Read the model definition and answer for the solid it produces. Units are mm, in the model's axes. A direction names the side the tool comes from. Coordinates: 2 decimals unless noted, no trailing zeros. Write each loop counter-clockwise with the first axis right and the second up, starting at its lowest first coordinate (ties: lowest second). Pieces come first, ordered by that corner, then holes. Notation, with made-up numbers: M 34.25,9 L 39.25,9 A16 cw 39.25,28 Z; hole C 41.25,-32.5 d4. An arc over 180 degrees is marked long. Use a Markdown table: item, result. Add a question column.
from build123d import *

# Parameters (mm, degrees)
SKETCH_1_W                  = 80
SKETCH_1_H                  = 83
EXTRUDE_1_DEPTH             = 12
HOLE_WIZARD_1_D             = 9
HOLE_WIZARD_1_CBORE_D       = 15
HOLE_WIZARD_1_CBORE_DEPTH   = 8
HOLE_WIZARD_1_2_D           = 46
HOLE_WIZARD_M6_2_D          = 5
HOLE_WIZARD_M6_1_AT_2_COUNT = 2
HOLE_WIZARD_M6_1_AT_2_PITCH = 15
CHAMFER_1_SIZE              = 1


with BuildPart() as part:
    # 草图1 → 凸台-拉伸1 (new body)
    with BuildSketch(Plane(origin=(0, 0, 0), x_dir=(0, 0, -1), z_dir=(1, 0, 0))):
        Rectangle(SKETCH_1_W, SKETCH_1_H)
    extrude(amount=EXTRUDE_1_DEPTH)

    # Hole Wizard 1 (through all)
    with Locations(Plane.ZY):
        with Locations((-25, 33.5), (25, 33.5)):
            CounterBoreHole(HOLE_WIZARD_1_D / 2, HOLE_WIZARD_1_CBORE_D / 2, HOLE_WIZARD_1_CBORE_DEPTH)

    # Hole Wizard 1 2 (through all)
    with Locations(Plane(origin=(12, 0, 0), x_dir=(0, 0, -1), z_dir=(1, 0, 0))):
        with Locations((0, -16.5)):
            Hole(HOLE_WIZARD_1_2_D / 2)

    # M6 螺纹孔2 (through all)
    with Locations(Plane.ZY):
        with Locations((-30, -16.5), (30, -16.5)):
            Hole(HOLE_WIZARD_M6_2_D / 2)

    # 草图8 → M6 螺纹孔1 (revolve, cut)
    with BuildSketch(Plane(origin=(6, -9, -40), x_dir=(0, 1, 0), z_dir=(1, 0, 0))):
        Polygon((0, 0), (0, 16.502151548), (2.5, 15), (2.5, 0), align=None)
    hole_wizard_m6_1 = revolve(axis=Axis((6, -9, -46.35), (0, 0, 1)), mode=Mode.SUBTRACT)

    # M6 螺纹孔1 at 2: M6 螺纹孔1 ×2
    with Locations(*[(0, -i * HOLE_WIZARD_M6_1_AT_2_PITCH, 0) for i in range(1, HOLE_WIZARD_M6_1_AT_2_COUNT)]):
        add(hole_wizard_m6_1, mode=Mode.SUBTRACT)

    # 镜向1: M6 螺纹孔1 across plane
    add(hole_wizard_m6_1.mirror(Plane.XY), mode=Mode.SUBTRACT)

    # 镜向1 copy 1 sketch → 镜向1 copy 1 (revolve, cut)
    with BuildSketch(Plane(origin=(6, -24, 40), x_dir=(0, 1, 0), z_dir=(1, 0, 0))):
        Polygon((0, 0), (0, -16.502151548), (2.5, -15), (2.5, 0), align=None)
    revolve(axis=Axis((6, -24, 46.35), (0, 0, 1)), mode=Mode.SUBTRACT)

    # 倒角1
    chamfer_1_edges = [part.edges().sort_by_distance(p)[0] for p in [
        (12, 41.5, 0),
    ]]
    chamfer(chamfer_1_edges, length=CHAMFER_1_SIZE)


solid = part.part
Item 1: Consider probe 1 along Y at (x, z) = (6, 35.5); probe 2 along Y at (x, z) = (6, -27.75); probe 3 along Y at (x, z) = (10.4, -25). Determine where each line is inside the solid, lowest interval first.
Item 2: Determine the mould class of faces 1 (the flat face through (6, -1, -40)), 2 (the flat face through (5, 41.5, 1)), 3 (the cylindrical face through (3.94, 26.18, 23.37)) for opening direction Y: pulls with the +Y half, pulls with the -Y half, needs draft (parallel to the pull), parting line crosses it, or undercut.
Item 3: For faces 4 (the cylindrical face through (4.31, -25.84, 32.61)), 5 (the cylindrical face through (4.31, -10.84, -32.61)), 6 (the flat face through (8, 34, -20)), determine the directions among +Z, -Z, +X, -X, +Y, -Y from which every point of the face is accessible in a straight line to the end or side of a thin tool.
Item 4: Find section B-B on y = 33.5. Give the vertices of the cut face in (x, z).
Item 5: Find section A-A on z = 0. Give the vertices of the cut face in (x, y), then the cut area to 4 significant figures.
Item 6: Find section C-C on y = -16.5. Give the vertices of the cut face in (x, z), then the cut area to 3 significant figures.
Item 7: Find section D-D on y = 1. Give the vertices of the cut face in (x, z).
Item 8: Each of these flat-tipped pins is pushed along its axis until it touches: pin 1 (10.5 mm diameter, centred on y = 33.5, z = -25, fed in from -X); pin 2 (6 mm diameter, centred on y = -16.5, z = -30, fed in from -X); pin 3 (4 mm diameter, centred on x = 6, y = -24, fed in from +Z); pin 4 (3 mm diameter, centred on x = 6, y = -9, fed in from -Z). Where does it stop, or does it pass through?
Geometry says:
| question | item | result |
|---|---|---|
| 1 | probe 1 | y = -41.5 to -26.5, -21.5 to -11.5, -6.5 to 41.5 |
| 1 | probe 2 | y = -41.5 to -26.5, -21.5 to -17.59, -15.41 to -11.5, -6.5 to 26.52, 40.48 to 41.5 |
| 1 | probe 3 | y = -41.5 to 29, 38 to 41.5 |
| 2 | face 1 | needs draft |
| 2 | face 2 | pulls with the +Y half |
| 2 | face 3 | undercut |
| 3 | face 4 | +Z |
| 3 | face 5 | -Z |
| 3 | face 6 | -X |
| 4 | outline | M 0,-40 L 12,-40 L 12,-29.5 L 8,-29.5 L 8,-32.5 L 0,-32.5 Z; M 0,-17.5 L 8,-17.5 L 8,-20.5 L 12,-20.5 L 12,20.5 L 8,20.5 L 8,17.5 L 0,17.5 Z; M 0,32.5 L 8,32.5 L 8,29.5 L 12,29.5 L 12,40 L 0,40 Z |
| 5 | outline | M 0,-41.5 L 12,-41.5 L 12,-39.5 L 0,-39.5 Z; M 0,6.5 L 12,6.5 L 12,40.5 L 11,41.5 L 0,41.5 Z |
| 5 | area | 443.5 mm2 |
| 6 | outline | M 0,-40 L 12,-40 L 12,-32.5 L 0,-32.5 Z; M 0,-27.5 L 12,-27.5 L 12,-23 L 0,-23 Z; M 0,23 L 12,23 L 12,27.5 L 0,27.5 Z; M 0,32.5 L 12,32.5 L 12,40 L 0,40 Z |
| 6 | area | 288 mm2 |
| 7 | outline | M 0,-40 L 12,-40 L 12,-14.92 L 0,-14.92 Z; M 0,14.92 L 12,14.92 L 12,40 L 0,40 Z |
| 8 | pin 1 | stops at x = 8 |
| 8 | pin 2 | stops at x = 0 |
| 8 | pin 3 | stops at z = 24.7 |
| 8 | pin 4 | stops at z = -24.4 |
